Read the model definition and answer for the solid it produces. Units are mm, in the model's axes. A direction names the side the tool comes from. Round coordinates to 2 decimals unless told otherwise and drop trailing zeros. Loops run counter-clockwise (first coordinate to the right, second up) from the corner with the lowest first, then second, coordinate; pieces in that order, holes last. Notation, with made-up numbers: M 73.5,29 L 103.5,29 A34 cw 103.5,68 Z; hole C -30.75,13.25 d3. An arc over 180 degrees is marked long. Write each question's results on one line, items separated by ' | '.
from build123d import *

# Parameters (mm, degrees)
CROQUIS1_W              = 42.2
CROQUIS1_H              = 10
SALIENTE_EXTRUIR1_DEPTH = 42
CROQUIS2_W              = 7.5
CROQUIS2_H              = 2.5
SALIENTE_EXTRUIR2_DEPTH = 5
CROQUIS3_R              = 11
CORTAR_EXTRUIR1_DEPTH   = 25


with BuildPart() as part:
    # Croquis1 → Saliente-Extruir1 (new body)
    with BuildSketch(Plane.XY):
        with Locations((21.1, -5)):
            Rectangle(CROQUIS1_W, CROQUIS1_H)
    extrude(amount=SALIENTE_EXTRUIR1_DEPTH)

    # Croquis2 → Saliente-Extruir2 (add)
    with BuildSketch(Plane.XY.offset(42)):
        with Locations((21.1, -5)):
            Rectangle(CROQUIS2_W, CROQUIS2_H)
    extrude(amount=SALIENTE_EXTRUIR2_DEPTH)

    # Croquis3 → Cortar-Extruir1 (cut)
    with BuildSketch(Plane(origin=(0, 0, 0), x_dir=(1, 0, 0), z_dir=(0, 1, 0))):
        with Locations(Location((21.1, -21, 0), (0, 0, 270))):
            Circle(CROQUIS3_R)
    extrude(amount=-CORTAR_EXTRUIR1_DEPTH, mode=Mode.SUBTRACT)


solid = part.part
Item 1: Flat-ended cylindrical pins translate along their axes: pin 1 (4 mm diameter, centred on x = 22, z = 45.5, fed in from +Y); pin 2 (6 mm diameter, centred on x = 21.5, y = -7, fed in from +Z); pin 3 (1.2 mm diameter, centred on y = -5.5, z = 45, fed in from +X); pin 4 (1.5 mm diameter, centred on x = 22.5, z = 45, fed in from -Y). Find the tip coordinate at first contact, or state that the pin passes through.
Outcome:
pin 1: stops at y = -3.75 | pin 2: stops at z = 47 | pin 3: stops at x = 24.85 | pin 4: stops at y = -6.25
Item 2: For faces 1 (the face through (21, -5, 47)), 2 (the face through (24.85, -5, 44)), 3 (the face through (21, -3.75, 44)), 4 (the face through (21, -6.25, 44)), 5 (the face through (17.35, -5, 44)), determine the directions among +Z, -Z, +X, -X, +Y, -Y from which every point of the face is accessible in a straight line to the end or side of a thin tool.
Outcome:
face 1: +Z, +X, -X, +Y, -Y | face 2: +Z, +X, +Y, -Y | face 3: +Z, +X, -X, +Y | face 4: +Z, +X, -X, -Y | face 5: +Z, -X, +Y, -Y
Item 3: The part is cut by section C-C (y = -5.25). Determine the outline of the cut face in (x, z).
Outcome:
outline: M 0,0 L 42.2,0 L 42.2,42 L 24.85,42 L 24.85,47 L 17.35,47 L 17.35,42 L 0,42 Z; hole C 21.1,21 d22
Item 4: The part is cut by section B-B (z = 21). Determine the outline of the cut face in (x, y).
Outcome:
outline: M 0,-10 L 10.1,-10 L 10.1,0 L 0,0 Z; M 32.1,-10 L 42.2,-10 L 42.2,0 L 32.1,0 Z
Item 5: The mould has two halves that part along X. Classify faces 6 (the face through (0, -5, 21)), 7 (the face through (30, -10, 30)), 8 (the face through (30.375, -4.93, 26.914)): pulls with the +X half, pulls with the -X half, needs draft (parallel to the pull), parting line crosses it, or undercut.
Outcome:
face 6: pulls with the -X half | face 7: needs draft | face 8: undercut
Item 6: The part is cut by section A-A (x = 21.1). Determine the outline of the cut face in (y, z), plus the area to 4 significant figures.
Outcome:
outline: M -10,0 L 0,0 L 0,10 L -10,10 Z; M -10,32 L 0,32 L 0,42 L -3.75,42 L -3.75,47 L -6.25,47 L -6.25,42 L -10,42 Z | area: 212.5 mm2
Item 7: Straight lines are drawn through the part: line 1 (X direction, y = -3.5, z = 21); line 2 (Z direction, x = 36, y = -1); line 3 (Z direction, x = 21, y = -6.75). For each, find the intervals that lie inside material, in ascending order.
Outcome:
line 1: x = 0 to 10.1, 32.1 to 42.2 | line 2: z = 0 to 42 | line 3: z = 0 to 10, 32 to 42
Item 8: The part is cut by section D-D (x = 14). Determine the outline of the cut face in (y, z).
Outcome:
outline: M -10,0 L 0,0 L 0,12.6 L -10,12.6 Z; M -10,29.4 L 0,29.4 L 0,42 L -10,42 Z
